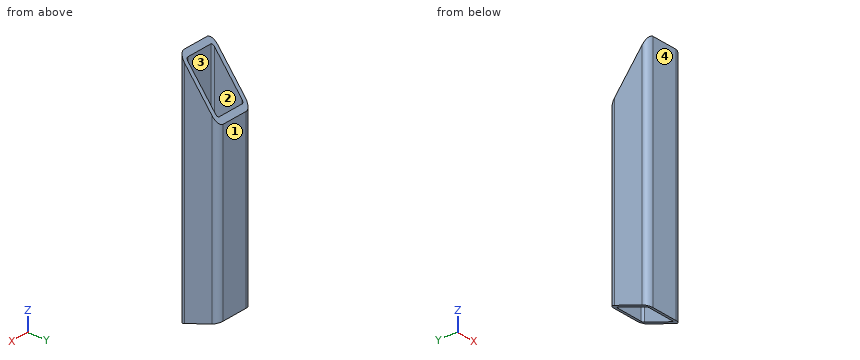
Autodesk Inventor part; units mm, degrees
ref_plane "Start Plane" through (0, 0, -3.4097) normal (0, 0, 1) x (1, 0, 0)
ref_plane "End Plane" through (0, 0, 117.2353) normal (0, 0, 1) x (1, 0, 0)
ref_plane "Work Plane4" through (-0.0634, -10.0438, -3.4033) normal (0.002, 0.3209, -0.9471) x (0.9999, -0.0123, -0.002)
ref_plane "Start Plane" through (0, 0, -3.4097) normal (0, 0, 1) x (1, 0, 0)
ref_plane "End Plane" through (0, 0, 117.2353) normal (0, 0, 1) x (1, 0, 0)
sketch "Sketch" plane through (0, 0, 0) normal (0, 0, 1) x (1, 0, 0)
  line L0 (-10, -7) -> (-10, 7)
  line L1 (-7, 10) -> (7, 10)
  line L2 (10, 7) -> (10, -7)
  line L3 (7, -10) -> (-7, -10)
  arc A0 (-10, -7) -> (-7, -10) centre (-7, -7) ccw
  arc A1 (-7, 10) -> (-10, 7) centre (-7, 7) ccw
  arc A2 (10, 7) -> (7, 10) centre (7, 7) ccw
  arc A3 (7, -10) -> (10, -7) centre (7, -7) ccw
  arc A4 (-7, 8) -> (-8, 7) centre (-7, 7) ccw
  line L4 (-7, 8) -> (7, 8)
  arc A5 (8, 7) -> (7, 8) centre (7, 7) ccw
  line L5 (8, 7) -> (8, -7)
  arc A6 (7, -8) -> (8, -7) centre (7, -7) ccw
  line L6 (7, -8) -> (-7, -8)
  arc A7 (-8, -7) -> (-7, -8) centre (-7, -7) ccw
  line L7 (-8, -7) -> (-8, 7)
  line L8 (0, 14.8698) -> (0, -14.8698) construction
  line L9 (-14.8698, 0) -> (14.8698, 0) construction
  dimension "d7" = 3
  dimension "d10" = 20
  dimension "d11" = 20
  dimension "d12" = 2
  dimension "d15" = 10
  dimension "d16" = 10
extrude "Body" add sketch "Sketch" along normal up to surface (120.6451 mm away) from surface at -3.4097
sketch "Sketch3" plane through (0, 0, 0) normal (0, 0, 1) x (1, 0, 0)
  line L0 (0, 0) -> (10, 0)
ref_plane "Work Plane3" through (0, 0, 0) normal (0, -1, 0) x (1, 0, 0)
sketch "Sketch4" plane through (0, 0, 0) normal (0, -1, 0) x (1, 0, 0)
  line L0 (-2, -3.4097) -> (12, -3.4097)
  line L1 (-2, 117.2353) -> (12, 117.2353)
  dimension "d18" = 120.645
ref_plane "Work Plane4" through (-0.0634, -10.0438, -3.4033) normal (0.002, 0.3209, -0.9471) x (0.9999, -0.0123, -0.002)
split "Split1" plane through (-0.0634, -10.0438, -3.4033) removes the side toward (0.002, 0.3209, -0.9471)
ref_plane "Work Plane5" through (219.4811, -4.3152, 110.7144) normal (-0.0027, 0.7958, 0.6055) x (1, 0.0014, 0.0027)
split "Split2" plane through (219.4811, -4.3152, 110.7144) removes the side toward (-0.0027, 0.7958, 0.6055)
ref_plane "Work Plane7" through (0.108, -1.8289, -14.111) normal (-0.0027, 0.7958, 0.6055) x (-1, -0.0023, -0.0016)
sketch "Sketch6" plane through (0.108, -1.8289, -14.111) normal (-0.0027, 0.7958, 0.6055) x (-1, -0.0023, -0.0016)
  circle A0 centre (-0.1219, -14.9734) radius 2.25
  circle A1 centre (-0.1219, -14.9734) radius 4
  point P0 (0.0818, 10.1227)
  dimension "d22" = 8
extrude "Extrusion2" [suppressed]
equation "\"d7\" = G_IR"
equation "\"d10\" = G_H"
equation "\"d11\" = G_W"
equation "\"d12\" = G_T"
equation "\"d15\" = 0.5 * d10"
equation "\"d16\" = 0.5 * d11"
equation "\"d3\" = G_L"
equation "\"G_W\" = 20"
equation "\"G_H\" = 20"
equation "\"G_T\" = 2"
equation "\"G_IR\" = 3"
equation "\"G_L\" = d18"
equation "\"G_OFFSET_START\" = 3.40974"
equation "\"G_OFFSET_END\" = 13.16879"
equation "\"d13\" = -G_OFFSET_START"
equation "\"d14\" = G_OFFSET_END + B_L"
equation "\"B_L\" = 104.06651"
properties part number "ISO 12633-2 - 20x20x2 - 120.65" material "Steel, Mild"
Read the model definition and answer for the solid it produces. Units are mm, in the model's axes. Face numbers are marked on the shaded views. Give positions to 0.01 mm unless a question says otherwise; leave off trailing zeros. Write each loop counter-clockwise with the first axis right and the second up, starting at its lowest first coordinate (ties: lowest second). Pieces come first, ordered by that corner, then holes. Notation, with made-up numbers: (1.5, 27.25) - (45.5, 27.25) arc R30 cw to (45.5, 54.25) - close; hole circle Ø10 at (-26, 46.25). An arc over 180 degrees is marked (long way). Write item = value, one per line. Start each with the question number.
Item 1: Find section C-C (x = -1.25). Give the vertices of the cut face in (y, z), then the cut area to 3 significant figures.
Item 2: Find section B-B (z = 33). Give the vertices of the cut face in (x, y).
Item 3: Find section D-D (z = 97). Give the vertices of the cut face in (x, y), then the cut area to 3 significant figures.
Item 4: The mould has two halves that part along Y. Classify the marked faces 1, 2, 3 and 4: +Y half, -Y half, draft (parallel to the pull), parting line (faces both ways), or undercut.
Item 5: Find section A-A (y = 3.75). Give the vertices of the cut face in (x, z), then the cut area to 3 significant figures.
Item 6: Find the intervals of material crossed by probe 1 along X at (y, z) = (1.5, 10); probe 2 along Y at (x, z) = (3, 103), in increasing order. Write a range as [from, to].
Item 7: This flat-tipped pin is pushed along its axis until it touches: P1, Ø4, axis at x = 5, z = 103, coming from the +Y side. Where does it stop, or does it pass through?
Response:
q1.outline = (-10, -3.39) - (-8, -2.71) - (-8, 114.57) - (-10, 117.2) - close; (8, 2.71) - (10, 3.39) - (10, 90.92) - (8, 93.54) - close
q1.area = 416 mm²
q2.outline = (-10, -7) arc R3 ccw to (-7, -10) - (7, -10) arc R3 ccw to (10, -7) - (10, 7) arc R3 ccw to (7, 10) - (-7, 10) arc R3 ccw to (-10, 7) - close; hole (-8, -7) arc R1 ccw to (-7, -8) - (7, -8) arc R1 ccw to (8, -7) - (8, 7) arc R1 ccw to (7, 8) - (-7, 8) arc R1 ccw to (-8, 7) - close
q3.outline = (-10, -7) arc R3 ccw to (-7, -10) - (7, -10) arc R3 ccw to (10, -7) - (10, 5.41) - (8, 5.4) - (8, -7) arc R1 cw to (7, -8) - (-7, -8) arc R1 cw to (-8, -7) - (-8, 5.35) - (-10, 5.34) - close
q3.area = 90.1 mm²
q4.face_1 = +Y half
q4.face_2 = undercut
q4.face_3 = undercut
q4.face_4 = -Y half
q5.outline = (-10, 1.25) - (-8, 1.25) - (-8, 99.1) - (-10, 99.09) - close; (8, 1.29) - (10, 1.29) - (10, 99.18) - (8, 99.17) - close
q5.area = 391 mm²
q6.probe_1 = [-10, -8], [8, 10]
q6.probe_2 = [-10, -8]
q7.P1 = -8
